Check sheet for the modelled part. Datum: model origin and axes. Units: mm. Round coordinates to 2 decimals unless told otherwise and drop trailing zeros. Write each loop counter-clockwise with the first axis right and the second up, starting at its lowest first coordinate (ties: lowest second). Pieces come first, ordered by that corner, then holes. Notation, with made-up numbers: (72, 75.5) -> (115, 75.5) arc R28 ccw to (115, 96.5) -> close; hole circle Ø6 at (-16, -19.5). An arc over 180 degrees is marked (long way). Use one line per item in the form item = value. Start each with the question number.
```python
from build123d import *

# Parameters (mm, degrees)
SKETCH_1_R          = 1.6
SKETCH_1_R_2        = 6.075
EXTRUDE_1_DEPTH     = 3
SKETCH_6_R          = 6.075
SKETCH_6_R_2        = 5.5
EXTRUDE_3_DEPTH     = 3
CUT_EXTRUDE_3_DEPTH = 10
EXTRUDE_4_DEPTH     = 3
CUT_EXTRUDE_4_DEPTH = 10
EXTRUDE_5_DEPTH     = 3
SKETCH_11_R         = 1.5
CUT_EXTRUDE_5_DEPTH = 10
SKETCH1_W           = 13.017216885
SKETCH1_H           = 13.916417238
CUT_EXTRUDE1_DEPTH  = 2
CHAMFER1_SIZE       = 10
FILLET1_R           = 10
FILLET2_R           = 3


with BuildPart() as part:
    # 草图1 → 凸台-拉伸1 (new body)
    with BuildSketch(Plane.XY.offset(4)):
        Polygon((27.5, -75), (27.5, -38.070079149), (27.5, 15), (-12.093715748, 15), (-12.093715748, -75), align=None)
        with Locations(Location((22.5, -12, 0), (0, 0, 180))):
            Circle(SKETCH_1_R, mode=Mode.SUBTRACT)
        with Locations(Location((22.5, -55, 0), (0, 0, 180))):
            Circle(SKETCH_1_R, mode=Mode.SUBTRACT)
        with Locations(Location((22.5, -67, 0), (0, 0, 180))):
            Circle(SKETCH_1_R, mode=Mode.SUBTRACT)
        with Locations(Location((-7.5, -67, 0), (0, 0, 180))):
            Circle(SKETCH_1_R, mode=Mode.SUBTRACT)
        with Locations(Location((-9.093715748, -18.5, 0), (0, 0, 180))):
            Circle(SKETCH_1_R, mode=Mode.SUBTRACT)
        with Locations(Location((0.406284252, 0, 0), (0, 0, 180))):
            Circle(SKETCH_1_R_2, mode=Mode.SUBTRACT)
        with Locations(Location((-9.093715748, -45.5, 0), (0, 0, 180))):
            Circle(SKETCH_1_R, mode=Mode.SUBTRACT)
    extrude(amount=-EXTRUDE_1_DEPTH)

    # 草图6 → 凸台-拉伸3 (add)
    with BuildSketch(Plane.XY.offset(4)):
        with Locations((0.406284252, 0)):
            Circle(SKETCH_6_R)
        with Locations((0.406284252, 0)):
            Circle(SKETCH_6_R_2, mode=Mode.SUBTRACT)
    extrude(amount=-EXTRUDE_3_DEPTH)

    # 草图7 → 切除-拉伸3 (cut)
    with BuildSketch(Plane.XY.offset(4)):
        with BuildLine():
            Line((16.573520953, -5.561905559), (-1.763823971, -11))
            ThreePointArc((-1.763823971, -11), (-2.785101184, -12.045663796), (-2.431704924, -13.463948325))
            Line((-2.431704924, -13.463948325), (15.90564, -33.025853884))
            ThreePointArc((15.90564, -33.025853884), (17.551570485, -33.394908599), (18.5, -32))
            Line((18.5, -32), (18.5, -7))
            ThreePointArc((18.5, -7), (17.897296336, -5.797977003), (16.573520953, -5.561905559))
        make_face()
        with BuildLine():
            Line((-4.093715748, -27.181985619), (-4.093715748, -52.572589617))
            ThreePointArc((-4.093715748, -52.572589617), (-3.190045848, -53.948958177), (-1.567861865, -53.666949617))
            Line((-1.567861865, -53.666949617), (11.100960059, -41.791186455))
            ThreePointArc((11.100960059, -41.791186455), (11.57432379, -40.745267595), (11.169466175, -39.670972572))
            Line((11.169466175, -39.670972572), (-1.499355748, -26.156131735))
            ThreePointArc((-1.499355748, -26.156131735), (-3.145286233, -25.78707702), (-4.093715748, -27.181985619))
        make_face()
        with BuildLine():
            Line((15.974146116, -48.188371256), (-1.326105415, -64.40564))
            ThreePointArc((-1.326105415, -64.40564), (-1.69516013, -66.051570485), (-0.300251531, -67))
            Line((-0.300251531, -67), (17, -67))
            ThreePointArc((17, -67), (18.060660172, -66.560660172), (18.5, -65.5))
            Line((18.5, -65.5), (18.5, -49.282731256))
            ThreePointArc((18.5, -49.282731256), (17.596330099, -47.906362696), (15.974146116, -48.188371256))
        make_face()
    extrude(amount=-CUT_EXTRUDE_3_DEPTH, mode=Mode.SUBTRACT)

    # 草图8 → 凸台-拉伸4 (add)
    with BuildSketch(Plane.XY.offset(4)):
        Polygon((-12.093715748, 15), (15.09823702, 15), (27.5, 15), (27.5, 35), (15.09823702, 35), (-12.093715748, 35), align=None)
    extrude(amount=-EXTRUDE_4_DEPTH)

    # 草图9 → 切除-拉伸4 (cut)
    with BuildSketch(Plane.XY.offset(4)):
        Polygon((27.5, 13.166002361), (27.5, 35), (9.950271794, 35), (-3.087828752, 35), (-12.093715748, 35), (-12.093715748, 24.5099793), (-12.093715748, 13.166002361), align=None)
    extrude(amount=-CUT_EXTRUDE_4_DEPTH, mode=Mode.SUBTRACT)

    # 草图10 → 凸台-拉伸5 (add)
    with BuildSketch(Plane.XY.offset(4)):
        Polygon((27.5, 13.166002361), (27.5, 2.997829135), (27.5, -1.956571947), (47.5, 14.825420677), (47.5, 22.166002361), (40.159418315, 22.166002361), (24.570961047, 13.166002361), align=None)
    extrude(amount=-EXTRUDE_5_DEPTH)

    # 草图11 → 切除-拉伸5 (cut)
    with BuildSketch(Plane.XY.offset(4)):
        with Locations((42.134580189, 16.938478334)):
            Circle(SKETCH_11_R)
    extrude(amount=-CUT_EXTRUDE_5_DEPTH, mode=Mode.SUBTRACT)

    # Sketch1 → Cut-Extrude1 (cut)
    with BuildSketch(Plane(origin=(47.5, 0, 0), x_dir=(0, 0, -1), z_dir=(1, 0, 0))):
        with Locations((-1.715406072, 17.791444366)):
            Rectangle(SKETCH1_W, SKETCH1_H)
    extrude(amount=-CUT_EXTRUDE1_DEPTH, mode=Mode.SUBTRACT)

    # Chamfer1
    chamfer1_edges = [part.edges().sort_by_distance(p)[0] for p in [
        (-12.093715748, 13.166002361, 2.5),
    ]]
    chamfer(chamfer1_edges, length=CHAMFER1_SIZE)

    # Fillet1
    fillet1_edges = [part.edges().sort_by_distance(p)[0] for p in [
        (27.5, -1.956571947, 2.5),
        (24.570961047, 13.166002361, 2.5),
    ]]
    fillet(fillet1_edges, radius=FILLET1_R)

    # Fillet2
    fillet2_edges = [part.edges().sort_by_distance(p)[0] for p in [
        (40.159418315, 22.166002361, 2.5),
        (45.5, 13.147221414, 2.5),
        (45.5, 22.166002361, 2.5),
    ]]
    fillet(fillet2_edges, radius=FILLET2_R)


solid = part.part
```
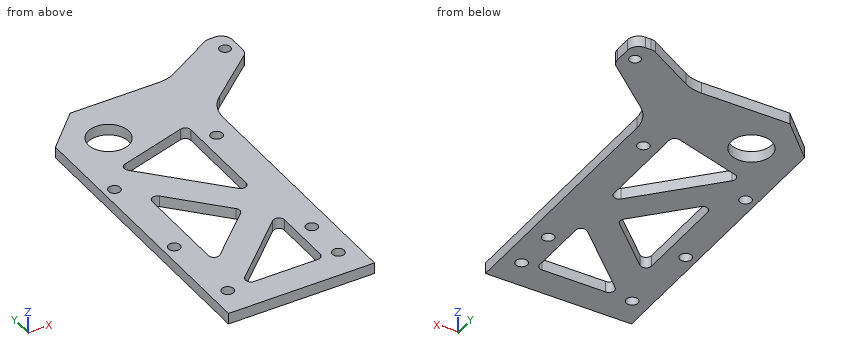
1. Sectioned sample at C-C (y = -55). Enter the section's corners in (x, z), and give its area (3 significant figures).
2. Sectioned sample at A-A (y = -18.5). Enter the section's corners in (x, z).
3. Scan lines: probe 1 along Y at (x, z) = (22.5, 1.8); probe 2 along Y at (x, z) = (-1, 3.75); probe 3 along Y at (x, z) = (-2, 1.3). Record each from-to range of solid material in increasing order.
4. Depth check by flat-ended pin: pin 1 (0.9 mm diameter, centred on y = -57.5, z = 2, fed in from +X); pin 2 (0.9 mm diameter, centred on x = 4, z = 3, fed in from +Y). Enter the tip coordinate at first touch or a pass-through.
5. Sectioned sample at B-B (z = 2.7). Give the number of separate pieces and of enclosed holes in the cut face, and give its area (3 significant figures).
6. Sectioned sample at D-D (x = 38). Enter the section's corners in (y, z), and give its area (3 significant figures).
Returned:
q1.outline = (-12.09, 1) -> (8.71, 1) -> (8.71, 4) -> (-12.09, 4) -> close; (18.5, 1) -> (20.9, 1) -> (20.9, 4) -> (18.5, 4) -> close; (24.1, 1) -> (27.5, 1) -> (27.5, 4) -> (24.1, 4) -> close
q1.area = 79.8 mm^2
q2.outline = (-12.09, 1) -> (-10.69, 1) -> (-10.69, 4) -> (-12.09, 4) -> close; (-7.49, 1) -> (2.29, 1) -> (2.29, 4) -> (-7.49, 4) -> close; (18.5, 1) -> (27.5, 1) -> (27.5, 4) -> (18.5, 4) -> close
q3.probe_1 = -75 to -68.6, -65.4 to -56.6, -53.4 to -13.6, -10.4 to 13.18
q3.probe_2 = -75 to -66.83, -64.1 to -53.13, -26.69 to -14.99, -10.77 to -5.32, 5.32 to 13.17
q3.probe_3 = -75 to -53.95, -25.8 to -13.92, -11.09 to -4.95, 4.95 to 13.17
q4.pin_1 = 27.5
q4.pin_2 = 13.17
q5.separate_pieces = 1
q5.enclosed_holes = 11
q5.area = 2,710 mm^2
q6.outline = (6.85, 1) -> (20.92, 1) -> (20.92, 4) -> (6.85, 4) -> close
q6.area = 42.2 mm^2
